from build123d import *

# Parameters (mm, degrees)
BOX406008011_W               = 17.5
BOX406008011_H               = 13.3
BOX406008011_DEPTH           = 19.7
BOX406008011_PLACEMENT_ANGLE = 20
BOX406008010_W               = 17.5
BOX406008010_H               = 13.3
BOX406008010_DEPTH           = 19.7
BOX406008010_PLACEMENT_ANGLE = 20
BOX406008007_W               = 18
BOX406008007_H               = 5.3
BOX406008007_DEPTH           = 14.9


with BuildPart() as cube346:
    # Box406008011 → Box406008011 (new body)
    with BuildSketch(Plane.XY):
        with Locations((8.75, 6.65)):
            Rectangle(BOX406008011_W, BOX406008011_H)
    extrude(amount=BOX406008011_DEPTH)


with BuildPart() as cube346_1:
    # Box406008011 placement: moved
    add(cube346.part.moved(Location((3.75, 6, 30.3))).rotate(Axis((3.75, 6, 30.3), (0, 1, 0)), BOX406008011_PLACEMENT_ANGLE))


with BuildPart() as part_mirroring:
    # Part__Mirroring: instance of Cube346
    add(cube346_1.part.mirror(Plane(origin=(0, 0, 0), x_dir=(0, -1, 0), z_dir=(1, 0, 0))))


with BuildPart() as fusion:
    # Box406008010 → Box406008010 (new body)
    with BuildSketch(Plane.XY):
        with Locations((8.75, 6.65)):
            Rectangle(BOX406008010_W, BOX406008010_H)
    extrude(amount=BOX406008010_DEPTH)


with BuildPart() as fusion_1:
    # Box406008010 placement: moved
    add(fusion.part.moved(Location((3.75, 6, 30.3))).rotate(Axis((3.75, 6, 30.3), (0, 1, 0)), BOX406008010_PLACEMENT_ANGLE))

    # Fusion: union Part__Mirroring
    add(part_mirroring.part)


with BuildPart() as obj1:
    # Box406008007 → Box406008007 (new body)
    with BuildSketch(Plane(origin=(-9, 13, 34.3), x_dir=(1, 0, 0), z_dir=(0, 0, 1))):
        with Locations((9, 2.65)):
            Rectangle(BOX406008007_W, BOX406008007_H)
    extrude(amount=BOX406008007_DEPTH)

    # Cut: cut Fusion
    add(fusion_1.part, mode=Mode.SUBTRACT)


with BuildPart() as obj1_1:
    # Cut placement: moved
    add(obj1.part.moved(Location((0, -1.5, -14))))


solid = obj1_1.part
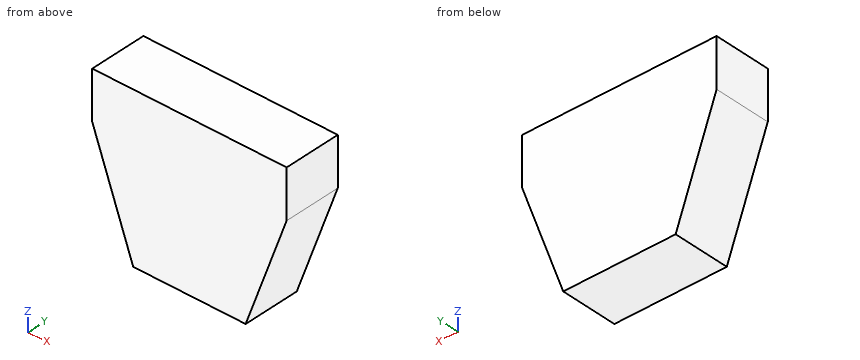
Design review of the part built by this model. Coordinates are the model's own, in mm. Coordinates: 2 decimals unless noted, no trailing zeros. Loops run counter-clockwise (first coordinate to the right, second up) from the corner with the lowest first, then second, coordinate; pieces in that order, holes last. Notation, with made-up numbers: (22, -40) -> (39, -40) arc R34 cw to (39, -2) -> close; hole circle Ø9 at (88.5, 30). An arc over 180 degrees is marked (long way). Use a Markdown table: item, result. Add a question column.
Item 1: Clearance check with a flat-ended pin moving along its axis: P1, Ø1, axis at y = 12.5, z = 27, coming from the -X side. State where the tip first meets the part, or that it passes through.
Item 2: We need section C-C, the plane z = 28. Write out the cut boundary in (x, y), and give its area (3 significant figures).
Item 3: Wall thickness on L1, parallel to X at y = 13.3, z = 29.5; L2, parallel to X at y = 15.35, z = 24: over which ranges is each line inside the solid? List them lowest first. Write a range as from..to.
Item 4: We need section A-A, the plane y = 12.3. Write out the cut boundary in (x, z), and give its area (3 significant figures).
Item 5: We need section B-B, the plane x = 8. Write out the cut boundary in (y, z).
Numbers:
| question | item | result |
|---|---|---|
| 1 | P1 | stops at x = -7.83 |
| 2 | outline | (-8.01, 11.5) -> (8.01, 11.5) -> (8.01, 16.8) -> (-8.01, 16.8) -> close |
| 2 | area | 84.9 mm^2 |
| 3 | L1 | x = -8.55..8.55 |
| 3 | L2 | x = -6.55..6.55 |
| 4 | outline | (-9, 30.72) -> (-5.21, 20.3) -> (5.21, 20.3) -> (9, 30.72) -> (9, 35.2) -> (-9, 35.2) -> close |
| 4 | area | 229 mm^2 |
| 5 | outline | (11.5, 27.98) -> (16.8, 27.98) -> (16.8, 35.2) -> (11.5, 35.2) -> close |
